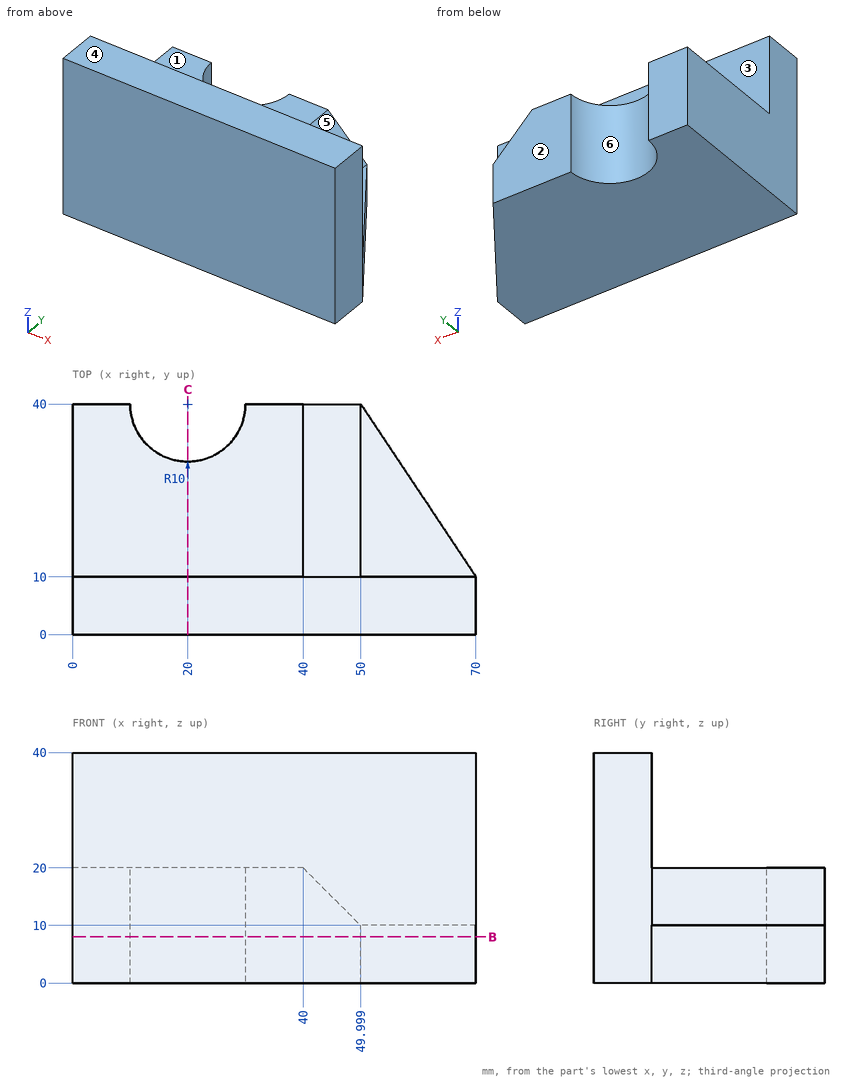
Drawing for the job (mm, zero at the part's lowest x, y, z). A direction names the side the tool comes from. Round coordinates to 2 decimals unless told otherwise and drop trailing zeros. Loops run counter-clockwise (first coordinate to the right, second up) from the corner with the lowest first, then second, coordinate; pieces in that order, holes last. Notation, with made-up numbers: (42.25, 41) -> (49.25, 41) arc R17 ccw to (49.25, 60) -> close; hole circle Ø3 at (-25.75, 80.25). An arc over 180 degrees is marked (long way). Use one line per item in the form item = value. Start each with the question number.
Item 1: Band-saw the part on C-C (x = 20). List the corners of the cut face in (y, z), plus the area to 3 significant figures.
Item 2: Band-saw the part on B-B (z = 8). List the corners of the cut face in (x, y).
Item 3: Tool access for the marked faces 1, 2 and 3: list every direction of +Z, -Z, +X, -X, +Y, -Y with a clear straight run to the whole face (end or side of a thin tool).
Item 4: Drill centre lines: line 1 along Y through (x, z) = (36.5, 27.5); line 2 along Z through (x, y) = (39, 35); line 3 along X through (y, z) = (37.5, 2.5) (1 decimal). Where is each one in solid material? Low to high.
Item 5: Two-plate mould, pull along X, no slides. Class the marked faces 4, 5 and 6: released by +X, released by -X, zero draft, split by the parting line, or undercut.
Item 6: Drop flat-ended pins along their axis: pin 1 Ø8 at (x, y) = (24, 16) entering from +Z; pin 2 Ø6 at (x, y) = (60, 24.5) entering from +Z; pin 3 Ø3 at (x, y) = (42.5, 24.5) entering from +Z. Give the stop position or say it passes through.
Data:
q1.outline = (0, 0) -> (30, 0) -> (30, 20) -> (10, 20) -> (10, 40) -> (0, 40) -> close
q1.area = 800 mm^2
q2.outline = (0, 0) -> (70, 0) -> (70, 10) -> (50, 40) -> (30, 40) arc R10 cw to (10, 40) -> (0, 40) -> close
q3.face_1 = +Z, +X, -X, +Y
q3.face_2 = +Z, -Z, +X, -X, +Y
q3.face_3 = +Z, +X, +Y
q4.line_1 = 0 to 10
q4.line_2 = 0 to 20
q4.line_3 = 0 to 10.3, 29.7 to 51.7
q5.face_4 = zero draft
q5.face_5 = released by +X
q5.face_6 = undercut
q6.pin_1 = 20
q6.pin_2 = 10
q6.pin_3 = 19
